Print and shaded views of the part. All mm, measured from the part's lowest x, y and z. A direction names the side the tool comes from. Give positions to 0.01 mm unless a question says otherwise; leave off trailing zeros. Loops run counter-clockwise (first coordinate to the right, second up) from the corner with the lowest first, then second, coordinate; pieces in that order, holes last. Notation, with made-up numbers: M 10,85 L 50,85 A29 ccw 50,108 Z; hole C -35,52 d2. An arc over 180 degrees is marked long. Answer as CSV lines item,"result".
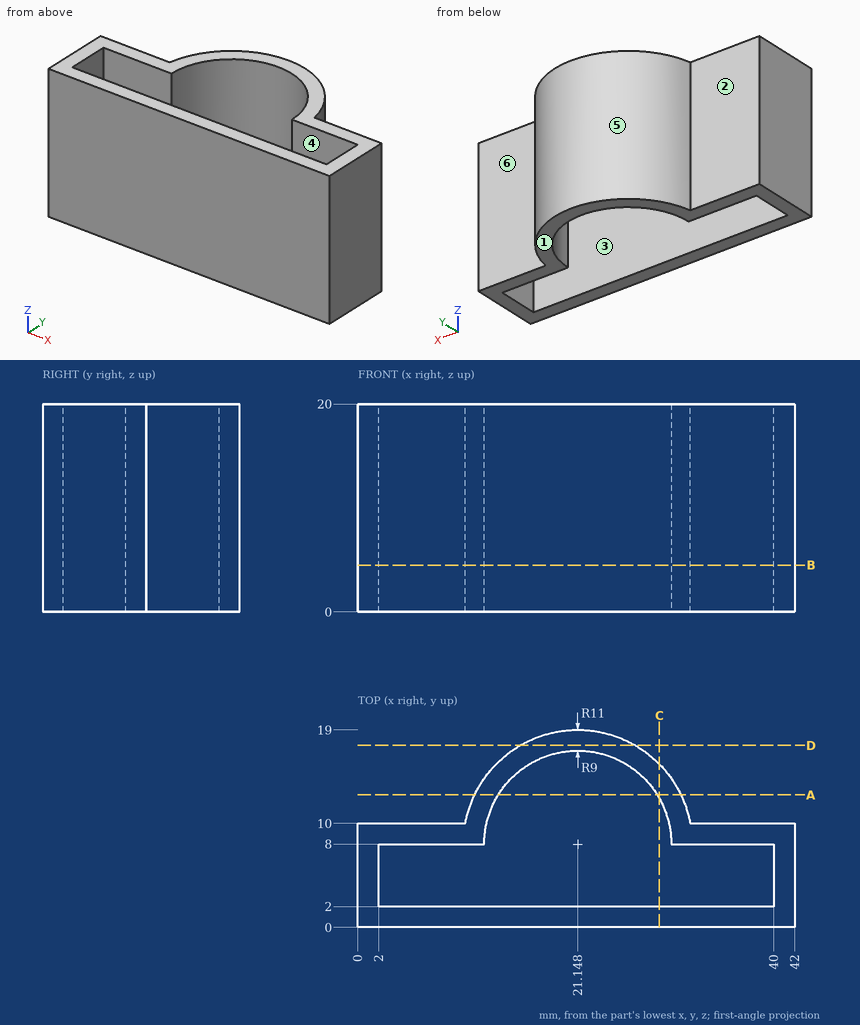
Q1. Cut at A-A (y = 12.75). Write the cut outline in (x, z).
Solution:
outline,"M 11.23,0 L 13.5,0 L 13.5,20 L 11.23,20 Z; M 28.79,0 L 31.07,0 L 31.07,20 L 28.79,20 Z"
Q2. Cut at C-C (x = 29). Write the cut outline in (y, z), and give its area (3 significant figures).
Solution:
outline,"M 0,0 L 2,0 L 2,20 L 0,20 Z; M 12.4,0 L 15.7,0 L 15.7,20 L 12.4,20 Z"
area,"106 mm²"
Q3. Wall check: line 1 (X direction, y = 3.25, z = 2.5); line 2 (Y direction, x = 9.5, z = 4.5); line 3 (X direction, y = 9.25, z = 9.5) (1 decimal). Give the ranges that are in metal, low to high. Write a range as [from, to].
Solution:
line 1,"x = [0, 2], [40, 42]"
line 2,"y = [0, 2], [8, 10]"
line 3,"x = [0, 12.2], [30.1, 42]"
Q4. Cut at B-B (z = 4.5). Write the cut outline in (x, y) (1 decimal).
Solution:
outline,"M 0,0 L 42,0 L 42,10 L 32,10 A11 ccw 10.3,10 L 0,10 Z; hole M 2,2 L 40,2 L 40,8 L 30.1,8 A9 ccw 12.1,8 L 2,8 Z"
Q5. Which spindle directions (+Z, -Z, +X, -X, +Y, -Y) get a long thin tool onto all of the face, cutting with end or side? Do the marked faces 1, 2 and 3. Say none if no direction does.
Solution:
face 1,"-Z, +X, -X, +Y, -Y"
face 2,"+Z, -Z, -X, +Y"
face 3,"+Z, -Z"
Q6. Cut at D-D (y = 17.5). Write the cut outline in (x, z), and give its area (3 significant figures).
Solution:
outline,"M 15.6,0 L 26.69,0 L 26.69,20 L 15.6,20 Z"
area,"222 mm²"
Q7. Mould opens along X. For the marked faces 4, 5 and 6 say: released by +X, released by -X, zero draft, split by the parting line, or undercut.
Solution:
face 4,"undercut"
face 5,"split by the parting line"
face 6,"zero draft"
Q8. Pin check, flat tips, straight feed: P1, Ø8, axis at x = 34.5, z = 8, coming from the +Y side; P2, Ø5, axis at x = 3.5, z = 6, coming from the +Y side; P3, Ø3, axis at x = 26.5, y = 13, coming from the -Z side; P4, Ø2, axis at x = 11, z = 3, coming from the +Y side. Stop position of each tip, or through.
Solution:
P1,"stops at y = 13.79"
P2,"stops at y = 10"
P3,"passes through"
P4,"stops at y = 14.11"
